```python
from build123d import *

# Parameters (mm, degrees)
BOSS_EXTRUDE1_DEPTH = 1.6
SKETCH2_R           = 1.4
CUT_EXTRUDE1_DEPTH  = 1.6


with BuildPart() as part:
    # Sketch1 → Boss-Extrude1 (new body)
    with BuildSketch(Plane.XY):
        with BuildLine():
            Line((48, -20), (-48, -20))
            ThreePointArc((-48, -20), (-49.414213562, -19.414213562), (-50, -18))
            Line((-50, -18), (-50, 18))
            ThreePointArc((-50, 18), (-49.414213562, 19.414213562), (-48, 20))
            Line((-48, 20), (48, 20))
            ThreePointArc((48, 20), (49.414213562, 19.414213562), (50, 18))
            Line((50, 18), (50, -18))
            ThreePointArc((50, -18), (49.414213562, -19.414213562), (48, -20))
        make_face()
    extrude(amount=BOSS_EXTRUDE1_DEPTH)

    # Sketch2 → Cut-Extrude1 (cut)
    with BuildSketch(Plane.XY.offset(1.6)):
        with Locations((-35, 11.75)):
            Circle(SKETCH2_R)
        with Locations(Location((-35, -11.75, 0), (0, 0, 180))):
            Circle(SKETCH2_R)
        with Locations((35, -11.75)):
            Circle(SKETCH2_R)
        with Locations(Location((35, 11.75, 0), (0, 0, 180))):
            Circle(SKETCH2_R)
        Polygon((23.5, 16.88), (-23.5, 16.88), (-28, 20), (28, 20), align=None)
        Polygon((28, -20), (23.5, -16.88), (-23.5, -16.88), (-28, -20), align=None)
    extrude(amount=-CUT_EXTRUDE1_DEPTH, mode=Mode.SUBTRACT)


solid = part.part
```
Check sheet for the modelled part. Datum: model origin and axes. Units: mm. A direction names the side the tool comes from. Give positions to 0.01 mm unless a question says otherwise; leave off trailing zeros. Order: outer loops, then holes, each group sorted by start corner. A loop starts at its lowest first (then second) coordinate and runs counter-clockwise, first axis right, second up. Notation, with made-up numbers: (82.25, -7.75) -> (127.25, -7.75) arc R18 ccw to (127.25, 14.25) -> close; hole circle Ø4 at (19.25, 69). An arc over 180 degrees is marked (long way). Return JSON: item names as keys, results as strings.
1. Cross-section at C-C, the plane z = 1.1. Record the cut outline in (x, y), plus the area to 3 significant figures.
From the geometry:
{"outline": "(-50, -18) arc R2 ccw to (-48, -20) -> (-28, -20) -> (-23.5, -16.88) -> (23.5, -16.88) -> (28, -20) -> (48, -20) arc R2 ccw to (50, -18) -> (50, 18) arc R2 ccw to (48, 20) -> (28, 20) -> (23.5, 16.88) -> (-23.5, 16.88) -> (-28, 20) -> (-48, 20) arc R2 ccw to (-50, 18) -> close; hole circle Ø2.8 at (-35, -11.75); hole circle Ø2.8 at (-35, 11.75); hole circle Ø2.8 at (35, -11.75); hole circle Ø2.8 at (35, 11.75)", "area": "3,650 mm^2"}
2. Go/stop test with flat-tipped pins: P1, Ø3, axis at x = -35, y = 11.75, coming from the -Z side; P2, Ø0.5, axis at x = -0.5, z = 0.5, coming from the +Y side; P3, Ø0.5, axis at x = -10.5, z = 1, coming from the -Y side. Record where each tip stops, or that it passes through.
From the geometry:
{"P1": "z = 0", "P2": "y = 16.88", "P3": "y = -16.88"}
3. Mould release check, pull along Y, two halves, no side actions. Record for faces 4 (the cylindrical face through (36.03, 10.8, 0.81)), 5 (the flat face through (-25.72, -18.42, 0.81)), 6 (the flat face through (25.78, 18.46, 0.81)): +Y half, -Y half, draft (parallel to the pull), parting line (faces both ways), or undercut.
From the geometry:
{"face 4": "undercut", "face 5": "-Y half", "face 6": "+Y half"}
4. Cross-section at D-D, the plane x = -1.5. Record the cut outline in (y, z), plus the area to 3 significant figures.
From the geometry:
{"outline": "(-16.88, 0) -> (16.88, 0) -> (16.88, 1.6) -> (-16.88, 1.6) -> close", "area": "54.0 mm^2"}
5. Cross-section at B-B, the plane y = 11.75. Record the cut outline in (x, z).
From the geometry:
{"outline": "(-50, 0) -> (-36.4, 0) -> (-36.4, 1.6) -> (-50, 1.6) -> close; (-33.6, 0) -> (33.6, 0) -> (33.6, 1.6) -> (-33.6, 1.6) -> close; (36.4, 0) -> (50, 0) -> (50, 1.6) -> (36.4, 1.6) -> close"}
6. Set-up check for faces 1 (the flat face through (25.78, -18.46, 0.81)), 2 (the cylindrical face through (-49.43, 19.4, 0.79)), 3 (the flat face through (-25.72, 18.42, 0.81)): record each of +Z, -Z, +X, -X, +Y, -Y from which the full face is reachable in a straight line by a thin tool's end or side.
From the geometry:
{"face 1": "+Z, -Z, -Y", "face 2": "+Z, -Z, -X, +Y", "face 3": "+Z, -Z, +Y"}
7. Material ranges on probe 1 along Y at (x, z) = (35, 0.75); probe 2 along Y at (x, z) = (36, 1.05); probe 3 along Y at (x, z) = (-3, 0.45), recorded low to high. Write a range as [from, to].
From the geometry:
{"probe 1": "[-20, -13.15], [-10.35, 10.35], [13.15, 20]", "probe 2": "[-20, -12.73], [-10.77, 10.77], [12.73, 20]", "probe 3": "[-16.88, 16.88]"}
8. Cross-section at A-A, the plane x = -35. Record the cut outline in (y, z).
From the geometry:
{"outline": "(-20, 0) -> (-13.15, 0) -> (-13.15, 1.6) -> (-20, 1.6) -> close; (-10.35, 0) -> (10.35, 0) -> (10.35, 1.6) -> (-10.35, 1.6) -> close; (13.15, 0) -> (20, 0) -> (20, 1.6) -> (13.15, 1.6) -> close"}
